Build history of the part. All positions in model axes, mm. Face numbers are marked on the shaded views. A direction names the side the tool comes from. Give positions to 0.01 mm unless a question says otherwise; leave off trailing zeros. Order: outer loops, then holes, each group sorted by start corner. A loop starts at its lowest first (then second) coordinate and runs counter-clockwise, first axis right, second up. Notation, with made-up numbers: (1, 31) -> (54, 31) arc R22 cw to (54, 39) -> close; hole circle Ø7 at (-32, 65.5). An arc over 180 degrees is marked (long way). One line per item, written item: value. Start each with the question number.
(1) Two-plate mould, pull along Z, no slides. Class the marked faces 1, 2, 3 and 4: +Z half, -Z half, draft (parallel to the pull), parting line (faces both ways), or undercut.
(2) Probe line 1 (Z direction, x = 15.5, y = 5.5); line 2 (Z direction, x = 25.25, y = 21.55); line 3 (X direction, y = 18.25, z = 4.5). List the from-to ranges inside material, lowest first.
(3) Which spindle directions (+Z, -Z, +X, -X, +Y, -Y) get a long thin tool onto all of the face, cutting with end or side? Do the marked faces 5, 6, 7 and 8. Say none if no direction does.
(4) Pin check, flat tips, straight feed: pin 1 (1.9 mm diameter, centred on x = 10, z = 17.5, fed in from +Y); pin 2 (0.8 mm diameter, centred on x = 18, y = 7.5, fed in from -Z); pin 3 (1.1 mm diameter, centred on y = 1, z = 12.5, fed in from +X). Stop position of each tip, or through.
(5) Saw through at A-A on y = 16.25. Give the cut face in (x, z).
(6) Saw through at B-B on z = 18. Give the cut face in (x, y), plus the area to 3 significant figures.
(7) Saw through at C-C on x = 25.25. Give the cut face in (y, z) (1 decimal).
(8) Saw through at D-D on z = 3. Give the cut face in (x, y), plus the area to 3 significant figures.
```python
from build123d import *

# Parameters (mm, degrees)
EXTRUDE_1_DEPTH     = 7
CUT_EXTRUDE_START   = -5
SKETCH_2_R          = 4
CUT_EXTRUDE_1_DEPTH = 5
SKETCH_3_W          = 29.5
SKETCH_3_H          = 11
EXTRUDE_2_DEPTH     = 8
SKETCH_4_W          = 7.5
SKETCH_4_H          = 10
SKETCH_4_W_2        = 10
EXTRUDE_3_DEPTH     = 7
SKETCH_5_W          = 9
SKETCH_5_H          = 9
CUT_EXTRUDE_2_DEPTH = 2
SKETCH_6_R          = 2.5
CUT_EXTRUDE_3_DEPTH = 2.2
SKETCH_7_R          = 1.6
CUT_EXTRUDE_4_DEPTH = 45.443784717
SKETCH_8_W          = 11.533749137
SKETCH_8_H          = 5
EXTRUDE_4_DEPTH     = 8
CUT_EXTRUDE_5_DEPTH = 3
SKETCH_11_W         = 8
SKETCH_11_H         = 6.5
EXTRUDE_6_DEPTH     = 5
EXTRUDE_7_DEPTH     = 1
EXTRUDE_8_DEPTH     = 1
CUT_EXTRUDE_6_DEPTH = 4
SKETCH_15_W         = 7
SKETCH_15_H         = 4.5
CUT_EXTRUDE_7_DEPTH = 2
SKETCH_16_W         = 1
SKETCH_16_H         = 4
CUT_EXTRUDE_8_DEPTH = 1


# Read off the part's stored shape, not the designer's step: 圆顶1, 圆顶2
with BuildPart() as part:
    # 草图1 → 凸台-拉伸1 (new body)
    with BuildSketch(Plane(origin=(0, 0, 0), x_dir=(1, 0, 0), z_dir=(0, 1, 0))):
        with BuildLine():
            Line((0, 0), (29.5, 0))
            Line((29.5, 0), (29.5, -2.5))
            Line((29.5, -2.5), (33.5, -2.5))
            ThreePointArc((33.5, -2.5), (37.5, -6.5), (33.5, -10.5))
            Line((33.5, -10.5), (29.5, -10.5))
            Line((29.5, -10.5), (29.5, -13))
            Line((29.5, -13), (0, -13))
            Line((0, -13), (0, -10.5))
            Line((0, -10.5), (-4, -10.5))
            ThreePointArc((-4, -10.5), (-8, -6.5), (-4, -2.5))
            Line((-4, -2.5), (0, -2.5))
            Line((0, -2.5), (0, 0))
        make_face()
    extrude(amount=EXTRUDE_1_DEPTH)

    # 草图2 → 切除-拉伸1 (cut)
    with BuildSketch(Plane(origin=(0, 7, 0), x_dir=(1, 0, 0), z_dir=(0, 1, 0)).offset(CUT_EXTRUDE_START)):
        with Locations((-4, -6.5)):
            Circle(SKETCH_2_R)
        with Locations((33.5, -6.5)):
            Circle(SKETCH_2_R)
    extrude(amount=CUT_EXTRUDE_1_DEPTH, mode=Mode.SUBTRACT)

    # 草图3 → 凸台-拉伸2 (add)
    with BuildSketch(Plane(origin=(0, 7, 0), x_dir=(1, 0, 0), z_dir=(0, 1, 0))):
        with Locations((14.75, -6.5)):
            Rectangle(SKETCH_3_W, SKETCH_3_H)
    extrude(amount=EXTRUDE_2_DEPTH)

    # 草图4 → 凸台-拉伸3 (add)
    with BuildSketch(Plane(origin=(0, 15, 0), x_dir=(1, 0, 0), z_dir=(0, 1, 0))):
        with Locations((25.25, -6.5)):
            Rectangle(SKETCH_4_W, SKETCH_4_H)
        with Locations((5.5, -6.5)):
            Rectangle(SKETCH_4_W_2, SKETCH_4_H)
    extrude(amount=EXTRUDE_3_DEPTH)

    # 草图5 → 切除-拉伸2 (cut)
    with BuildSketch(Plane(origin=(0, 22, 0), x_dir=(1, 0, 0), z_dir=(0, 1, 0))):
        with Locations((5.5, -6.5)):
            Rectangle(SKETCH_5_W, SKETCH_5_H)
    extrude(amount=-CUT_EXTRUDE_2_DEPTH, mode=Mode.SUBTRACT)

    # 草图6 → 切除-拉伸3 (cut)
    with BuildSketch(Plane(origin=(0, 22, 0), x_dir=(1, 0, 0), z_dir=(0, 1, 0))):
        with Locations(Location((25.25, -6.5, 0), (0, 0, 270))):
            Circle(SKETCH_6_R)
        with Locations(Location((4.253331237, -6.5, 0), (0, 0, 270))):
            Circle(SKETCH_6_R)
    extrude(amount=-CUT_EXTRUDE_3_DEPTH, mode=Mode.SUBTRACT)

    # 圆顶1 outline → 圆顶1 (revolve)
    with BuildSketch(Plane(origin=(4.253331237, 0, 6.5), x_dir=(1, 0, 0), z_dir=(0, 0, 1))):
        with BuildLine():
            Line((0, 19.8), (2.500000001, 19.799999998))
            ThreePointArc((2.500000001, 19.799999998), (1.60078106, 21.238476323), (0, 21.8))
            Line((0, 21.8), (0, 19.8))
        make_face()
    revolve(axis=Axis((4.253331237, 0, 6.5), (0, 1, 0)))

    # 圆顶2 outline → 圆顶2 (revolve)
    with BuildSketch(Plane(origin=(25.25, 0, 6.5), x_dir=(1, 0, 0), z_dir=(0, 0, 1))):
        with BuildLine():
            Line((0, 19.8), (2.500000001, 19.799999997))
            ThreePointArc((2.500000001, 19.799999997), (1.60078106, 21.238476323), (0, 21.8))
            Line((0, 21.8), (0, 19.8))
        make_face()
    revolve(axis=Axis((25.25, 0, 6.5), (0, 1, 0)))

    # 草图7 → 切除-拉伸4 (cut, through all)
    with BuildSketch(Plane(origin=(0, 2, 0), x_dir=(1, 0, 0), z_dir=(0, 1, 0))):
        with Locations(Location((-4, -6.5, 0), (0, 0, 270))):
            Circle(SKETCH_7_R)
        with Locations(Location((33.5, -6.5, 0), (0, 0, 270))):
            Circle(SKETCH_7_R)
    extrude(amount=-CUT_EXTRUDE_4_DEPTH, mode=Mode.SUBTRACT)

    # 草图8 → 凸台-拉伸4 (add)
    with BuildSketch(Plane.XY.offset(13)):
        with Locations((14.355989937, 2.5)):
            Rectangle(SKETCH_8_W, SKETCH_8_H)
    extrude(amount=EXTRUDE_4_DEPTH)

    # 草图10 → 切除-拉伸5 (cut)
    with BuildSketch(Plane.XZ):
        Polygon((8.589115368, 21), (8.589115368, 12), (1, 12), (1, 1), (28.5, 1), (28.5, 12), (20.122864505, 12), (20.122864505, 21), align=None)
    extrude(amount=-CUT_EXTRUDE_5_DEPTH, mode=Mode.SUBTRACT)

    # 草图11 → 凸台-拉伸6 (add)
    with BuildSketch(Plane(origin=(0, 5, 0), x_dir=(1, 0, 0), z_dir=(0, 1, 0))):
        with Locations((14.355989936, -17.75)):
            Rectangle(SKETCH_11_W, SKETCH_11_H)
    extrude(amount=EXTRUDE_6_DEPTH)

    # 草图12 → 凸台-拉伸7 (add)
    with BuildSketch(Plane(origin=(18.355989936, 0, 0), x_dir=(0, 0, -1), z_dir=(1, 0, 0))):
        Polygon((-14.5, 8.832927064), (-13, 8.172497524), (-13, 5), (-14.5, 5), align=None)
    extrude(amount=-EXTRUDE_7_DEPTH)

    # 草图13 → 凸台-拉伸8 (add)
    with BuildSketch(Plane.ZY.offset(-10.355989936)):
        Polygon((14.5, 8.832927064), (13, 8.172497524), (13, 5), (14.5, 5), align=None)
    extrude(amount=-EXTRUDE_8_DEPTH)

    # 草图14 → 切除-拉伸6 (cut)
    with BuildSketch(Plane.XY.offset(21)):
        Polygon((10.855989936, 5), (17.855989936, 5), (17.855989936, 9.5), (15.355989936, 9.5), (15.355989936, 10), (13.355989936, 10), (13.355989936, 9.5), (10.855989936, 9.5), align=None)
    extrude(amount=-CUT_EXTRUDE_6_DEPTH, mode=Mode.SUBTRACT)

    # 草图15 → 切除-拉伸7 (cut)
    with BuildSketch(Plane.XY.offset(17)):
        with Locations((14.355989936, 7.25)):
            Rectangle(SKETCH_15_W, SKETCH_15_H)
    extrude(amount=-CUT_EXTRUDE_7_DEPTH, mode=Mode.SUBTRACT)

    # 草图16 → 切除-拉伸8 (cut)
    with BuildSketch(Plane(origin=(0, 10, 0), x_dir=(1, 0, 0), z_dir=(0, 1, 0))):
        with Locations((11.355989936, -16.5)):
            Rectangle(SKETCH_16_W, SKETCH_16_H)
        with Locations((17.355989936, -16.5)):
            Rectangle(SKETCH_16_W, SKETCH_16_H)
    extrude(amount=-CUT_EXTRUDE_8_DEPTH, mode=Mode.SUBTRACT)


solid = part.part
```
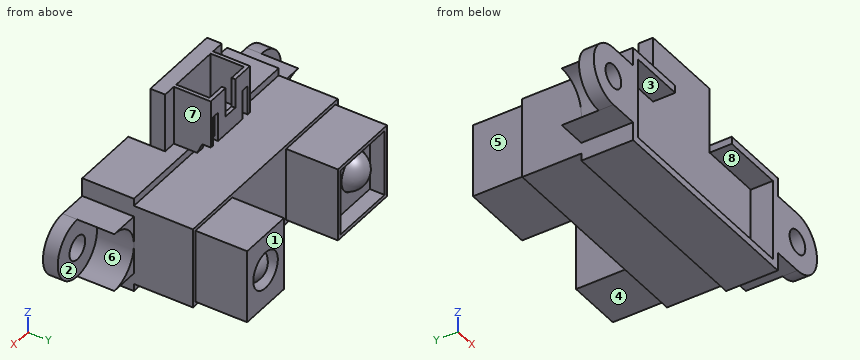
Results below:
1. face 1: draft
1. face 2: undercut
1. face 3: undercut
1. face 4: -Z half
2. line 1: z = 0 to 13, 14.5 to 15
2. line 2: z = 1.5 to 4, 5.4 to 7.6, 9 to 11.5
2. line 3: x = 0.5 to 10.5, 21.5 to 29
3. face 5: +Z, -Z, -X, +Y
3. face 6: +X, +Y
3. face 7: +Z, +X, +Y
3. face 8: -Y
4. pin 1: stops at y = 10
4. pin 2: stops at z = 1
4. pin 3: stops at x = 29.5
5. outline: (0.5, 1.5) -> (10.5, 1.5) -> (10.5, 11.5) -> (0.5, 11.5) -> close; (21.5, 1.5) -> (29, 1.5) -> (29, 11.5) -> (21.5, 11.5) -> close
6. outline: (8.59, 3) -> (20.12, 3) -> (20.12, 5) -> (18.36, 5) -> (18.36, 10) -> (17.86, 10) -> (17.86, 5) -> (10.86, 5) -> (10.86, 10) -> (10.36, 10) -> (10.36, 5) -> (8.59, 5) -> close; (11.86, 9.5) -> (13.36, 9.5) -> (13.36, 10) -> (11.86, 10) -> close; (15.36, 9.5) -> (16.86, 9.5) -> (16.86, 10) -> (15.36, 10) -> close
6. area: 29.6 mm²
7. outline: (0, 0) -> (7, 0) -> (7, 1) -> (15, 1) -> (15, 1.5) -> (22, 1.5) -> (22, 4) -> (19.8, 4) arc R2.6 ccw to (19.8, 9) -> (22, 9) -> (22, 11.5) -> (15, 11.5) -> (15, 12) -> (7, 12) -> (7, 13) -> (0, 13) -> (0, 12) -> (3, 12) -> (3, 1) -> (0, 1) -> close
8. outline: (-5.94, 0) -> (1, 0) -> (1, 3) -> (28.5, 3) -> (28.5, 0) -> (35.44, 0) -> (35.44, 2) -> (31.56, 2) -> (31.56, 7) -> (29.5, 7) -> (29.5, 15) -> (29, 15) -> (29, 22) -> (21.5, 22) -> (21.5, 15) -> (10.5, 15) -> (10.5, 22) -> (10, 22) -> (10, 20) -> (1, 20) -> (1, 22) -> (0.5, 22) -> (0.5, 15) -> (0, 15) -> (0, 7) -> (-2.06, 7) -> (-2.06, 2) -> (-5.94, 2) -> close
8. area: 509 mm²
